Read the model definition and answer for the solid it produces. Units are mm, in the model's axes. Face numbers are marked on the shaded views. Coordinates: 2 decimals unless noted, no trailing zeros. Loops run counter-clockwise (first coordinate to the right, second up) from the corner with the lowest first, then second, coordinate; pieces in that order, holes last. Notation, with made-up numbers: (51.25, 60.5) -> (79.25, 60.5) arc R30 ccw to (79.25, 85.5) -> close; hole circle Ø2 at (62, 18.25). An arc over 180 degrees is marked (long way). Answer as a JSON object with one key per item and string values. Group by question number.
1) Section C-C, the plane y = -8.75 is taken. Give the vertices of the cut face in (x, z).
2) Consider probe 1 along Y at (x, z) = (0, 1.7); probe 2 along X at (y, z) = (0.5, 1.2); probe 3 along X at (y, z) = (16.5, 1.15). Determine where each line is inside the solid, lowest interval first. Write a range as [from, to].
3) Section A-A, the plane x = 0 is taken. Give the vertices of the cut face in (y, z), plus the area to 3 significant figures.
4) Section B-B, the plane x = 15.5 is taken. Give the vertices of the cut face in (y, z).
5) Determine the mould class of the marked faces 1, 2 and 3 for opening direction Y: released by +Y, released by -Y, zero draft, split by the parting line, or undercut.
6) A flat-ended cylindrical pin translates along its axis: P1, Ø1.5, axis at y = 14, z = 2, coming from the +X side. Find the tip coordinate at first contact, or state that the pin passes through.
7) Section D-D, the plane y = 11 is taken. Give the vertices of the cut face in (x, z), plus the area to 3 significant figures.
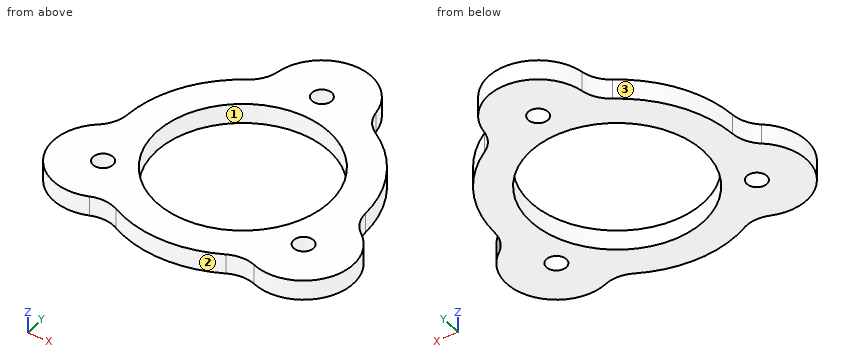
from build123d import *

# Parameters (mm, degrees)
SKETCH_2_R               = 8.75
EXTRUDE_1_DEPTH          = 3
SKETCH_3_R               = 1.5
CUT_EXTRUDE_1_DEPTH      = 34.87136207
PATTERN_CIRCULAR_1_COUNT = 3
PATTERN_CIRCULAR_1_ANGLE = 240
SKETCH_4_R               = 18
EXTRUDE_2_DEPTH          = 3
FILLET_1_R               = 5
SKETCH_5_R               = 13
CUT_EXTRUDE_2_DEPTH      = 34.87136222
SKETCH_6_R               = 1.5
CUT_EXTRUDE_3_DEPTH      = 34.87136222
PATTERN_CIRCULAR_2_COUNT = 3
PATTERN_CIRCULAR_2_ANGLE = 240


with BuildPart() as part:
    # 草图2 → 凸台-拉伸1 (new body)
    with BuildSketch(Plane.XY):
        with BuildLine():
            ThreePointArc((11.405444566, -15.245190528), (21.650635095, -12.5), (18.905444566, -2.254809472))
            ThreePointArc((18.905444566, -2.254809472), (10.556079661, 6.094555434), (7.5, 17.5))
            ThreePointArc((7.5, 17.5), (0, 25), (-7.5, 17.5))
            ThreePointArc((-7.5, 17.5), (-10.556079661, 6.094555434), (-18.905444566, -2.254809472))
            ThreePointArc((-18.905444566, -2.254809472), (-21.650635095, -12.5), (-11.405444566, -15.245190528))
            ThreePointArc((-11.405444566, -15.245190528), (0, -12.189110868), (11.405444566, -15.245190528))
        make_face()
        Circle(SKETCH_2_R, mode=Mode.SUBTRACT)
    extrude(amount=EXTRUDE_1_DEPTH)

    # 草图3 → 切除-拉伸1 (cut, through all)
    with BuildSketch(Plane.XY.offset(3)):
        with Locations((0, 17.5)):
            Circle(SKETCH_3_R)
    cut_extrude_1 = extrude(amount=-CUT_EXTRUDE_1_DEPTH, mode=Mode.SUBTRACT)

    # 阵列(圆周)1: 切除-拉伸1 ×3 about axis
    pattern_circular_1_axis = Axis((0, 0, 0), (0, 0, -1))
    for i in range(1, PATTERN_CIRCULAR_1_COUNT):
        add(cut_extrude_1.rotate(pattern_circular_1_axis, i * PATTERN_CIRCULAR_1_ANGLE / (PATTERN_CIRCULAR_1_COUNT - 1)), mode=Mode.SUBTRACT)

    # 草图4 → 凸台-拉伸2 (add)
    with BuildSketch(Plane.XY.offset(3)):
        Circle(SKETCH_4_R)
    extrude(amount=-EXTRUDE_2_DEPTH)

    # 圆角1
    fillet_1_edges = [part.edges().sort_by_distance(p)[0] for p in [
        (17.923796485, -1.65454512, 1.5),
        (7.529020137, 16.349735649, 1.5),
        (-7.529020137, 16.349735649, 1.5),
        (-17.923796485, -1.65454512, 1.5),
        (-10.394776348, -14.695190528, 1.5),
        (10.394776348, -14.695190528, 1.5),
    ]]
    fillet(fillet_1_edges, radius=FILLET_1_R)

    # 草图5 → 切除-拉伸2 (cut, through all)
    with BuildSketch(Plane.XY.offset(3)):
        Circle(SKETCH_5_R)
    extrude(amount=-CUT_EXTRUDE_2_DEPTH, mode=Mode.SUBTRACT)

    # 草图6 → 切除-拉伸3 (cut, through all)
    with BuildSketch(Plane.XY.offset(3)):
        with Locations((0, 17.5)):
            Circle(SKETCH_6_R)
    extrude(amount=-CUT_EXTRUDE_3_DEPTH, mode=Mode.SUBTRACT)

    # 阵列(圆周)2: 切除-拉伸1 ×3 about axis
    pattern_circular_2_axis = Axis((0, 0, -50.911688245), (0, 0, 1))
    for i in range(1, PATTERN_CIRCULAR_2_COUNT):
        add(cut_extrude_1.rotate(pattern_circular_2_axis, i * PATTERN_CIRCULAR_2_ANGLE / (PATTERN_CIRCULAR_2_COUNT - 1)), mode=Mode.SUBTRACT)


solid = part.part
Determined:
{
 "1": {"outline": "(-22.66, 0) -> (-16.66, 0) -> (-16.66, 3) -> (-22.66, 3) -> close; (-13.66, 0) -> (-9.61, 0) -> (-9.61, 3) -> (-13.66, 3) -> close; (9.61, 0) -> (13.66, 0) -> (13.66, 3) -> (9.61, 3) -> close; (16.66, 0) -> (22.66, 0) -> (22.66, 3) -> (16.66, 3) -> close"},
 "2": {"probe 1": "[-18, -13], [13, 16], [19, 25]", "probe 2": "[-18, -12.99], [12.99, 18]", "probe 3": "[-8.28, -1.12], [1.12, 8.28]"},
 "3": {"outline": "(-18, 0) -> (-13, 0) -> (-13, 3) -> (-18, 3) -> close; (13, 0) -> (16, 0) -> (16, 3) -> (13, 3) -> close; (19, 0) -> (25, 0) -> (25, 3) -> (19, 3) -> close", "area": "42.0 mm²"},
 "4": {"outline": "(-16.24, 0) -> (-10.21, 0) -> (-10.21, 3) -> (-16.24, 3) -> close; (-7.29, 0) -> (9.15, 0) -> (9.15, 3) -> (-7.29, 3) -> close"},
 "5": {"face 1": "undercut", "face 2": "released by -Y", "face 3": "released by +Y"},
 "6": {"P1": "x = 12.18"},
 "7": {"outline": "(-14.25, 0) -> (-6.93, 0) -> (-6.93, 3) -> (-14.25, 3) -> close; (6.93, 0) -> (14.25, 0) -> (14.25, 3) -> (6.93, 3) -> close", "area": "43.9 mm²"}
}
